Can you work these out from the model? Positions are in its coordinate system, mm. A direction names the side the tool comes from. Round coordinates to 2 decimals unless told otherwise and drop trailing zeros. Loops run counter-clockwise (first coordinate to the right, second up) from the corner with the lowest first, then second, coordinate; pieces in that order, holes last. Notation, with made-up numbers: (55.25, 21.25) -> (72.25, 21.25) arc R25 ccw to (72.25, 40.25) -> close; hole circle Ø10 at (-6, 84.25). An arc over 180 degrees is marked (long way). Use a Markdown table: item, result.
from build123d import *

# Parameters (mm, degrees)
SKETCH1_W           = 4
SKETCH1_H           = 26
BOSS_EXTRUDE1_DEPTH = 30
SKETCH2_R           = 4
CUT_EXTRUDE1_DEPTH  = 30


with BuildPart() as part:
    # Sketch1 → Boss-Extrude1 (new body)
    with BuildSketch(Plane.XY):
        Polygon((-17.861271676, 18.222543353), (12.138728324, 18.222543353), (12.138728324, -11.777456647), (-17.861271676, -11.777456647), (-17.861271676, -9.777456647), (4.138728324, -9.777456647), (4.138728324, 16.222543353), (-17.861271676, 16.222543353), align=None)
        with Locations((8.138728324, 3.222543353)):
            Rectangle(SKETCH1_W, SKETCH1_H, mode=Mode.SUBTRACT)
    extrude(amount=BOSS_EXTRUDE1_DEPTH)

    # Sketch2 → Cut-Extrude1 (cut)
    with BuildSketch(Plane(origin=(12.138728324, 0, 0), x_dir=(0, 0, -1), z_dir=(1, 0, 0))):
        with Locations((-15, 3.222543353)):
            Circle(SKETCH2_R)
    extrude(amount=-CUT_EXTRUDE1_DEPTH, mode=Mode.SUBTRACT)


solid = part.part
1. I want a section at D-D (z = 8.25). Please give me the cut outline in (x, y).
Answer sheet:
| item | result |
|---|---|
| outline | (-17.86, -11.78) -> (12.14, -11.78) -> (12.14, 18.22) -> (-17.86, 18.22) -> (-17.86, 16.22) -> (4.14, 16.22) -> (4.14, -9.78) -> (-17.86, -9.78) -> close; hole (6.14, -9.78) -> (10.14, -9.78) -> (10.14, 16.22) -> (6.14, 16.22) -> close |
2. I need wall thicknesses on line 1 (Y direction, x = 11.35, z = 15); line 2 (X direction, y = 0, z = 19.75); line 3 (Y direction, x = -13, z = 8.5). Which ranges of each line are inside material? Lowest first, please.
Answer sheet:
| item | result |
|---|---|
| line 1 | y = -11.78 to -0.78, 7.22 to 18.22 |
| line 2 | x = 4.14 to 6.14, 10.14 to 12.14 |
| line 3 | y = -11.78 to -9.78, 16.22 to 18.22 |
3. Which directions (+Z, -Z, +X, -X, +Y, -Y) give clear straight access to the entire face, cutting with the end or side of a thin tool? Please do faces 1 (the flat face through (4.139, 0, 18)), 2 (the flat face through (10.139, 0, 18)), 3 (the flat face through (5, 2, 0)).
Answer sheet:
| item | result |
|---|---|
| face 1 | +Z, -Z, -X |
| face 2 | +Z, -Z |
| face 3 | -Z, +X, -X, +Y, -Y |
4. Will this pin go through, and if not, where does the flat tip stop? pin 1 Ø1 at (y, z) = (6, 4.5) entering from -X.
Answer sheet:
| item | result |
|---|---|
| pin 1 | stops at x = 4.14 |
5. If we mould it in two halves opening along Y, with no side actions, what happens to faces 4 (the flat face through (12.139, 7, 18)), 5 (the flat face through (8, 16.223, 15)), 6 (the flat face through (8, -9.777, 15)), 7 (the flat face through (-3, 18.223, 15))? For each: +Y half, -Y half, draft (parallel to the pull), parting line (faces both ways), or undercut.
Answer sheet:
| item | result |
|---|---|
| face 4 | draft |
| face 5 | undercut |
| face 6 | undercut |
| face 7 | +Y half |
6. I want a section at A-A (y = 13). Please give me the cut outline in (x, z).
Answer sheet:
| item | result |
|---|---|
| outline | (4.14, 0) -> (6.14, 0) -> (6.14, 30) -> (4.14, 30) -> close; (10.14, 0) -> (12.14, 0) -> (12.14, 30) -> (10.14, 30) -> close |
7. I want a section at C-C (z = 15). Please give me the cut outline in (x, y), plus the area to 3 significant figures.
Answer sheet:
| item | result |
|---|---|
| outline | (-17.86, -11.78) -> (12.14, -11.78) -> (12.14, -0.78) -> (10.14, -0.78) -> (10.14, -9.78) -> (6.14, -9.78) -> (6.14, -0.78) -> (4.14, -0.78) -> (4.14, -9.78) -> (-17.86, -9.78) -> close; (-17.86, 16.22) -> (4.14, 16.22) -> (4.14, 7.22) -> (6.14, 7.22) -> (6.14, 16.22) -> (10.14, 16.22) -> (10.14, 7.22) -> (12.14, 7.22) -> (12.14, 18.22) -> (-17.86, 18.22) -> close |
| area | 192 mm² |
8. I want a section at B-B (x = -1.5). Please give me the cut outline in (y, z).
Answer sheet:
| item | result |
|---|---|
| outline | (-11.78, 0) -> (-9.78, 0) -> (-9.78, 30) -> (-11.78, 30) -> close; (16.22, 0) -> (18.22, 0) -> (18.22, 30) -> (16.22, 30) -> close |
